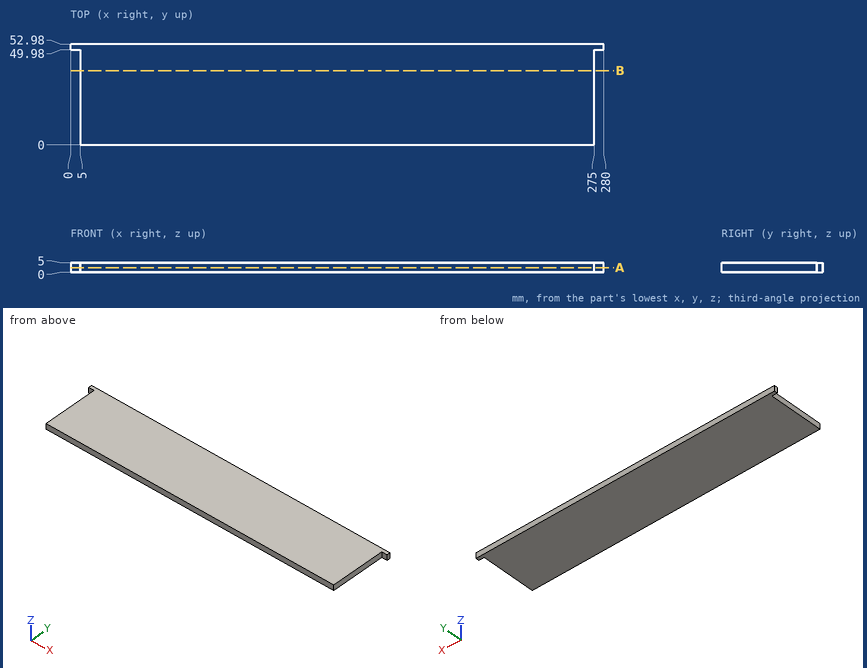
Part print with two shaded views. Sizes in mm from the minimum x, y, z corner. Give positions to 0.01 mm unless a question says otherwise; leave off trailing zeros. Order: outer loops, then holes, each group sorted by start corner. A loop starts at its lowest first (then second) coordinate and runs counter-clockwise, first axis right, second up. Notation, with made-up numbers: M 64.5,60.25 L 113.5,60.25 A15 ccw 113.5,77.25 Z; hole C -3,52.25 d9. An arc over 180 degrees is marked long. Use one line per item in the form item = value.
1) Probe probe 1 along X at (y, z) = (9.5, 3.9). List the from-to ranges inside material, lowest first.
Calculated:
probe_1 = 5 to 275
2) Saw through at A-A (z = 2.5). Give the cut face in (x, y).
Calculated:
outline = M 0,49.98 L 5,49.98 L 5,0 L 275,0 L 275,49.98 L 280,49.98 L 280,52.98 L 0,52.98 Z
3) Drop flat-ended pins along their axis: pin 1 (1.5 mm diameter, centred on x = 278, z = 3.5, fed in from -Y); pin 2 (1.5 mm diameter, centred on y = 26, z = 0.5, fed in from -X). Give the stop position or say it passes through.
Calculated:
pin_1 = 49.98
pin_2 = 5
4) Saw through at B-B (y = 39). Give the cut face in (x, z), plus the area to 3 significant figures.
Calculated:
outline = M 5,0 L 275,0 L 275,5 L 5,5 Z
area = 1,350 mm2
